Here's how the part is built. I have some questions about the finished solid (model axes, mm). Face numbers are marked on the shaded views. A direction names the side the tool comes from. Give positions to 0.01 mm unless a question says otherwise; leave off trailing zeros. Write each loop counter-clockwise with the first axis right and the second up, starting at its lowest first coordinate (ties: lowest second). Pieces come first, ordered by that corner, then holes. Notation, with made-up numbers: (84.5, 4.5) -> (88.5, 4.5) arc R19 ccw to (88.5, 9.5) -> close; hole circle Ø5 at (-22, 70.25). An arc over 180 degrees is marked (long way). Use CSV: the item, a comma, the result in double quotes. Start each with the question number.
(1) If we mould it in two halves opening along Y, with no side actions, what happens to the marked faces 4, 5 and 6? For each: pulls with the +Y half, pulls with the -Y half, needs draft (parallel to the pull), parting line crosses it, or undercut.
(2) Suppose I cut it at D-D on z = 2.8. List the corners of the cut face in (x, y) for me.
(3) I need wall thicknesses on L1, parallel to Y at x = 0, z = 3.2; L2, parallel to X at y = 0.8, z = 1; L3, parallel to Y at x = -0.35, z = 3.65. Which ranges of each line are inside material? Lowest first, please. Write a range as [from, to].
(4) Suppose I cut it at C-C on z = 1.6. List the corners of the cut face in (x, y) for me (3 decimals), plus the area to 3 significant figures.
(5) Suppose I cut it at A-A on x = 0. List the corners of the cut face in (y, z) for me (3 decimals).
(6) Which directions (+Z, -Z, +X, -X, +Y, -Y) give clear straight access to the entire face, cutting with the end or side of a thin tool? Please do the marked faces 1, 2 and 3.
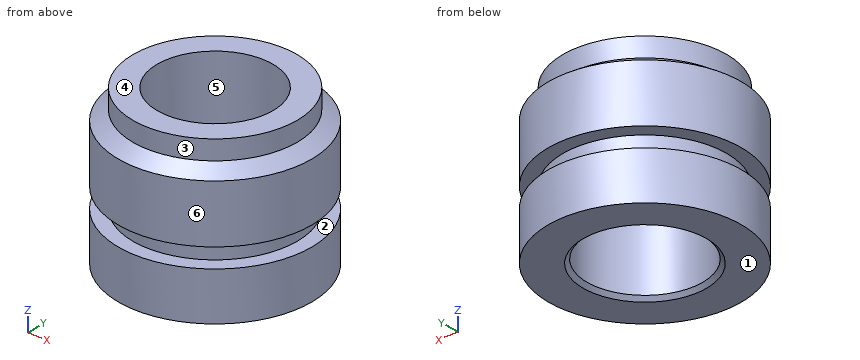
from build123d import *

# Parameters (mm, degrees)
SKETCH1_R           = 2.5
BOSS_EXTRUDE1_DEPTH = 4
SKETCH3_R           = 1.5
CUT_EXTRUDE1_DEPTH  = 5
CHAMFER1_SIZE       = 0.1


with BuildPart() as part:
    # Sketch1 → Boss-Extrude1 (new body)
    with BuildSketch(Plane.XY):
        Circle(SKETCH1_R)
    extrude(amount=BOSS_EXTRUDE1_DEPTH)

    # Sketch2 → Cut-Revolve1 (revolve, cut)
    with BuildSketch(Plane(origin=(0, 0, 0), x_dir=(1, 0, 0), z_dir=(0, 1, 0)), mode=Mode.PRIVATE) as cut_revolve1_sk:
        Polygon((-2.125, -4), (-3, -4), (-3, 0), (-2.5, 0), (-2.5, -1.25), (-2.125, -1.25), (-2.125, -1.75), (-2.5, -1.75), (-2.5, -3.25), (-2.125, -3.5), align=None)
    revolve(cut_revolve1_sk.sketch.rotate(Axis((0, 0, 4), (0, 0, -1)), 180), axis=Axis((0, 0, 4), (0, 0, -1)), mode=Mode.SUBTRACT)

    # Sketch3 → Cut-Extrude1 (cut)
    with BuildSketch(Plane(origin=(0, 0, 0), x_dir=(-1, 0, 0), z_dir=(0, 0, -1))):
        Circle(SKETCH3_R)
    extrude(amount=-CUT_EXTRUDE1_DEPTH, mode=Mode.SUBTRACT)

    # Chamfer1
    chamfer1_edges = [part.edges().sort_by_distance(p)[0] for p in [
        (1.5, 0, 0),
    ]]
    chamfer(chamfer1_edges, length=CHAMFER1_SIZE)


solid = part.part
Geometry says:
1,face 4,"needs draft"
1,face 5,"undercut"
1,face 6,"parting line crosses it"
2,outline,"circle Ø5 at (0, 0); hole circle Ø3 at (0, 0)"
3,L1,"[-2.5, -1.5], [1.5, 2.5]"
3,L2,"[-2.37, -1.27], [1.27, 2.37]"
3,L3,"[-2.1, -1.46], [1.46, 2.1]"
4,outline,"circle Ø4.25 at (0, 0); hole circle Ø3 at (0, 0)"
4,area,"7.12 mm²"
5,outline,"(-2.5, 0) -> (-1.6, 0) -> (-1.5, 0.1) -> (-1.5, 4) -> (-2.125, 4) -> (-2.125, 3.5) -> (-2.5, 3.25) -> (-2.5, 1.75) -> (-2.125, 1.75) -> (-2.125, 1.25) -> (-2.5, 1.25) -> close; (1.5, 0.1) -> (1.6, 0) -> (2.5, 0) -> (2.5, 1.25) -> (2.125, 1.25) -> (2.125, 1.75) -> (2.5, 1.75) -> (2.5, 3.25) -> (2.125, 3.5) -> (2.125, 4) -> (1.5, 4) -> close"
6,face 1,"-Z, +X, -X, +Y, -Y"
6,face 2,"none"
6,face 3,"+Z"
